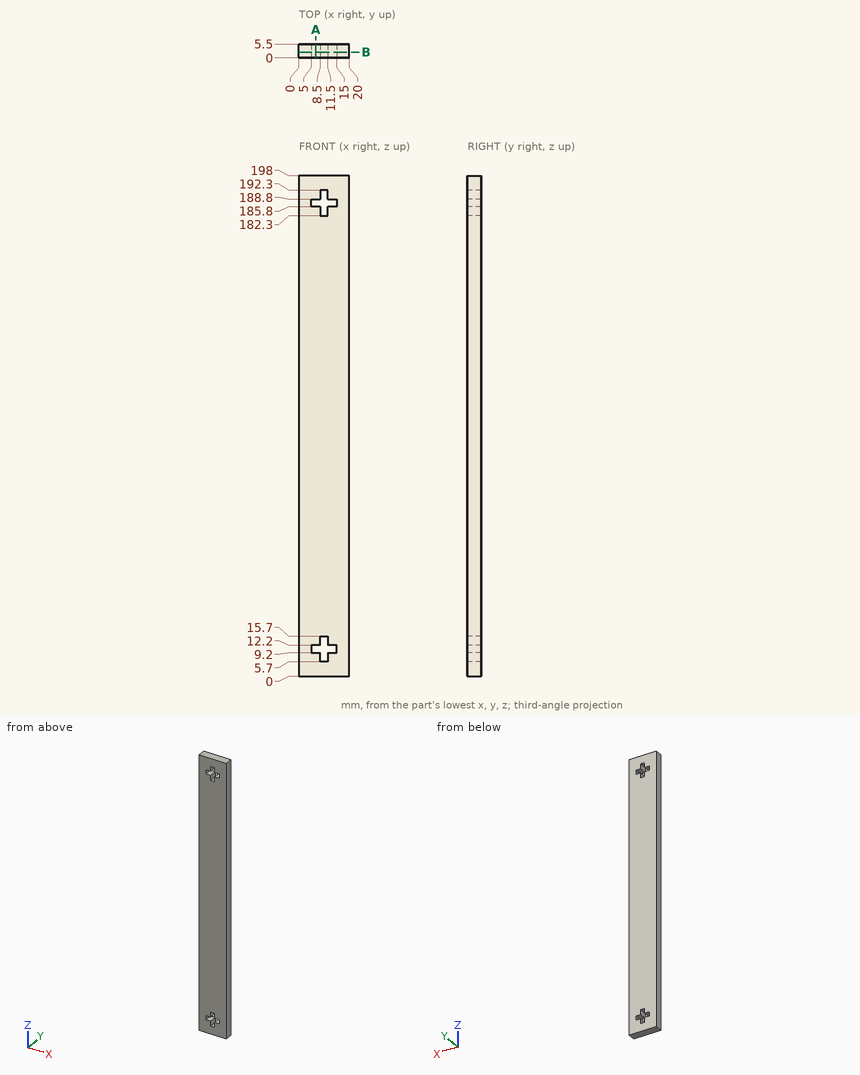
Geometry: see drawing. Coordinates: mm, zero at the bounding-box minimum. Coordinates: 2 decimals unless noted, no trailing zeros. Write each loop counter-clockwise with the first axis right and the second up, starting at its lowest first coordinate (ties: lowest second). Pieces come first, ordered by that corner, then holes.
1) Section A-A on x = 6.75. Output: boundary loops of the cut face in (y, z).
2) Material intervals for line 1 along Z through (x, y) = (10.25, 1); line 2 along Z through (x, y) = (8, 1.4); line 3 along X through (y, z) = (2.05, 10.5), sorted ascending.
3) Section B-B on y = 2.25. Output: boundary loops of the cut face in (x, z).
Check result:
1. outline: (0, 0) - (5.5, 0) - (5.5, 9.2) - (0, 9.2) - close; (0, 12.2) - (5.5, 12.2) - (5.5, 185.8) - (0, 185.8) - close; (0, 188.8) - (5.5, 188.8) - (5.5, 198) - (0, 198) - close
2. line 1: z = 0 to 5.7, 15.7 to 182.3, 192.3 to 198
2. line 2: z = 0 to 9.2, 12.2 to 185.8, 188.8 to 198
2. line 3: x = 0 to 5, 15 to 20
3. outline: (0, 0) - (20, 0) - (20, 198) - (0, 198) - close; hole (5, 9.2) - (8.5, 9.2) - (8.5, 5.7) - (11.5, 5.7) - (11.5, 9.2) - (15, 9.2) - (15, 12.2) - (11.5, 12.2) - (11.5, 15.7) - (8.5, 15.7) - (8.5, 12.2) - (5, 12.2) - close; hole (5, 185.8) - (8.5, 185.8) - (8.5, 182.3) - (11.5, 182.3) - (11.5, 185.8) - (15, 185.8) - (15, 188.8) - (11.5, 188.8) - (11.5, 192.3) - (8.5, 192.3) - (8.5, 188.8) - (5, 188.8) - close
